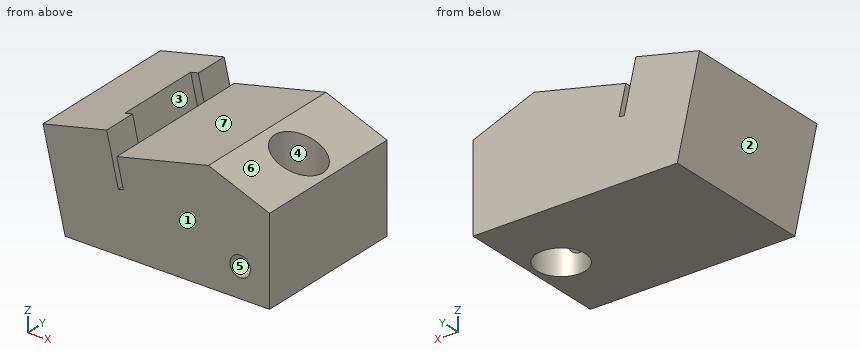
from build123d import *

# Parameters (mm, degrees)
F1_DEPTH = 15.175
F2_R     = 4.75
F3_DEPTH = 21.601
F4_W     = 1.54
F4_H     = 17
F5_DEPTH = 10
F6_R     = 2
F7_DEPTH = 10.8675781151


with BuildPart() as f1:
    # F0 (on Front) → F1 (new body, symmetric)
    with BuildSketch(Plane.XZ):
        Polygon((-20, 0), (20, 0), (20, 17), (8.0444113487, 21.6), (-9.9007201474, 17.3794053198), (-8.6173364513, 11.9227123817), (-9.5907752539, 11.6937650133), (-11.8802489381, 21.4281530397), (-24.35, 18.4953372502), align=None)
    extrude(amount=F1_DEPTH, both=True)

    # F2 (on face) → F3 (cut, through all)
    with BuildSketch(Plane(origin=(0, 0, 0), x_dir=(1, 0, 0), z_dir=(0, 0, -1))):
        with Locations((14.25, 0)):
            Circle(F2_R)
    extrude(amount=-F3_DEPTH, mode=Mode.SUBTRACT)

    # F4 (on face) → F5 (cut)
    with BuildSketch(Plane(origin=(-5.3983379501, 0, 22.9526622939), x_dir=(0.9734388026, 0, 0.2289473684), z_dir=(-0.2289473684, 0, 0.9734388026))):
        with Locations((-7.4287760529, 0)):
            Rectangle(F4_W, F4_H)
    extrude(amount=-F5_DEPTH, mode=Mode.SUBTRACT)

    # F6 (on face) → F7 (cut, through all)
    with BuildSketch(Plane.XZ.offset(15.175)):
        with Locations((14.25, 5.75)):
            Circle(F6_R)
    extrude(amount=-F7_DEPTH, mode=Mode.SUBTRACT)


solid = f1.part
Read the model definition and answer for the solid it produces. Units are mm, in the model's axes. Face numbers are marked on the shaded views. A direction names the side the tool comes from. Give positions to 0.01 mm unless a question says otherwise; leave off trailing zeros. Write each loop counter-clockwise with the first axis right and the second up, starting at its lowest first coordinate (ties: lowest second). Pieces come first, ordered by that corner, then holes. Notation, with made-up numbers: (39.5, -9.75) -> (95.5, -9.75) arc R18 ccw to (95.5, 12.25) -> close; hole circle Ø3 at (18.25, 1). An arc over 180 degrees is marked (long way). Answer as a JSON object with one key per item and string values. Group by question number.
1) The mould has two halves that part along Y. Classify the marked faces 1, 2, 3 and 4: +Y half, -Y half, draft (parallel to the pull), parting line (faces both ways), or undercut.
2) Find section C-C (z = 15.25). Write down the section's boundary in (x, y) (3 decimals).
3) Find section D-D (y = 0). Write down the section's boundary in (x, z).
4) Find section A-A (y = -7). Write down the section's boundary in (x, z).
5) A tool of negligible diameter and unlimited length cuts with its end or side. For the marked faces 5, 6 and 7, from which of +Z, -Z, +X, -X, +Y, -Y can it reach the whole face along a straight path? Write none if from no direction.
6) Consider L1, parallel to X at y = 0, z = 12.75; L2, parallel to Y at x = -12, z = 17.75 (3 decimals); L3, parallel to Y at x = 14.25, z = 12.5 (3 decimals). Determine where each line is inside the solid, lowest interval first. Write a range as from..to.
7) Each of these flat-tipped pins is pushed along its axis until it touches: P1, Ø1.5, axis at y = 1.5, z = 12.5, coming from the -X side; P2, Ø10, axis at y = 4, z = 9.5, coming from the -X side. Where does it stop, or does it pass through?
8) Find section B-B (x = 14.25). Write down the section's boundary in (y, z) (3 decimals).
Values follow:
{
 "1": {"face 1": "-Y half", "face 2": "draft", "face 3": "undercut", "face 4": "undercut"},
 "2": {"outline": "(-23.587, -15.175) -> (-10.427, -15.175) -> (-10.427, -8.5) -> (-12.009, -8.5) -> (-12.009, 8.5) -> (-10.427, 8.5) -> (-10.427, 15.175) -> (-23.587, 15.175) -> close; (-9.4, -15.175) -> (20, -15.175) -> (20, 15.175) -> (-9.4, 15.175) -> close; hole circle Ø9.5 at (14.25, 0)"},
 "3": {"outline": "(-24.35, 18.5) -> (-20, 0) -> (9.5, 0) -> (9.5, 21.04) -> (8.04, 21.6) -> (-9.9, 17.38) -> (-8.62, 11.92) -> (-11.09, 11.34) -> (-13.38, 21.08) -> close; (19, 0) -> (20, 0) -> (20, 17) -> (19, 17.38) -> close"},
 "4": {"outline": "(-24.35, 18.5) -> (-20, 0) -> (20, 0) -> (20, 17) -> (8.04, 21.6) -> (-9.9, 17.38) -> (-8.62, 11.92) -> (-11.09, 11.34) -> (-13.38, 21.08) -> close; hole circle Ø4 at (14.25, 5.75)"},
 "5": {"face 5": "-Y", "face 6": "+Z, +X, +Y, -Y", "face 7": "+Z, +Y, -Y"},
 "6": {"L1": "x = -23..-11.42, -8.81..9.5, 19..20", "L2": "y = -15.175..-8.5, 8.5..15.175", "L3": "y = -15.175..-4.75, 4.75..15.175"},
 "7": {"P1": "stops at x = -23.12", "P2": "stops at x = -23.41"},
 "8": {"outline": "(-15.175, 0) -> (-4.75, 0) -> (-4.75, 3.75) -> (-15.175, 3.75) -> close; (-15.175, 7.75) -> (-4.75, 7.75) -> (-4.75, 19.212) -> (-15.175, 19.212) -> close; (4.75, 0) -> (15.175, 0) -> (15.175, 19.212) -> (4.75, 19.212) -> close"}
}
